Work out the finished part from the listing and answer in its coordinate system (mm). Face numbers are marked on the shaded views. A direction names the side the tool comes from. Give positions to 0.01 mm unless a question says otherwise; leave off trailing zeros. Loops run counter-clockwise (first coordinate to the right, second up) from the corner with the lowest first, then second, coordinate; pieces in that order, holes last. Notation, with made-up numbers: M 89.25,3 L 101.25,3 A18 ccw 101.25,16 Z; hole C 27,-21 d9. An arc over 180 degrees is marked long. Write item = value, one per line. Start each with the question number.
1. Consider L1, parallel to Z at x = 2, y = 57; L2, parallel to Y at x = 2, z = -19; L3, parallel to X at y = 14, z = -28. Determine where each line is inside the solid, lowest interval first. Write a range as [from, to].
2. Flat-ended cylindrical pins translate along their axes: pin 1 Ø5 at (y, z) = (19.05, -19.05) entering from -X; pin 2 Ø4 at (x, z) = (6, -10.5) entering from +Y; pin 3 Ø11 at (y, z) = (57.15, -19.05) entering from +X; pin 4 Ø1 at (y, z) = (23.5, 15.5) entering from +X. Find the tip coordinate at first contact, or state that the pin passes through.
3. Section C-C on z = 19.05 is taken. Give the number of separate pieces and of enclosed holes in the cut face, plus the area to 3 significant figures.
4. For the marked faces 1, 2 and 3, determine the directions among +Z, -Z, +X, -X, +Y, -Y from which every point of the face is accessible in a straight line to the end or side of a thin tool.
5. The mould has two halves that part along Z. Classify the marked faces 4, 5 and 6: released by +Z, released by -Z, zero draft, split by the parting line, or undercut.
6. Section A-A on x = 19 is taken. Determine the outline of the cut face in (y, z).
```python
from build123d import *

# Parameters (mm, degrees)
BOSS_EXTRUDE1_DEPTH = 35.687
FILLET1_R           = 6.35
CUT_EXTRUDE1_REACH  = 94.367
SKETCH4_R           = 4.1656
CUT_EXTRUDE2_DEPTH  = 93.366725481


with BuildPart() as part:
    # Sketch2 → Boss-Extrude1 (new, symmetric)
    with BuildSketch(Plane.XY):
        with BuildLine():
            Line((0, 0), (0, 76.2))
            Line((0, 76.2), (6.35, 76.2))
            Line((6.35, 76.2), (6.35, 14.2748))
            ThreePointArc((6.35, 14.2748), (8.67112018, 8.67112018), (14.2748, 6.35))
            Line((14.2748, 6.35), (38.1, 6.35))
            Line((38.1, 6.35), (38.1, 0))
            Line((38.1, 0), (0, 0))
        make_face()
    extrude(amount=BOSS_EXTRUDE1_DEPTH, both=True)

    # Fillet1
    fillet1_edges = [part.edges().sort_by_distance(p)[0] for p in [
        (38.1, 6.35, 0),
        (6.35, 76.2, 0),
    ]]
    fillet(fillet1_edges, radius=FILLET1_R - 0.0001)  # a hair under: the kernel refuses the full size

    # Sketch3 → Cut-Extrude1 (cut, up to next)
    with BuildSketch(Plane.XZ, mode=Mode.PRIVATE) as cut_extrude1_sk1:
        with BuildLine():
            Line((25.4, 14.8844), (12.7, 14.8844))
            ThreePointArc((12.7, 14.8844), (8.5344, 19.05), (12.7, 23.2156))
            Line((12.7, 23.2156), (25.4, 23.2156))
            ThreePointArc((25.4, 23.2156), (29.5656, 19.05), (25.4, 14.8844))
        make_face()
    cut_extrude1_tool1 = extrude(cut_extrude1_sk1.sketch, amount=-CUT_EXTRUDE1_REACH, mode=Mode.PRIVATE) & part.part
    # Sketch3 → Cut-Extrude1 (cut, up to next)
    with BuildSketch(Plane.XZ, mode=Mode.PRIVATE) as cut_extrude1_sk2:
        with BuildLine():
            Line((25.4, -23.2156), (12.7, -23.2156))
            ThreePointArc((12.7, -23.2156), (8.5344, -19.05), (12.7, -14.8844))
            Line((12.7, -14.8844), (25.4, -14.8844))
            ThreePointArc((25.4, -14.8844), (29.5656, -19.05), (25.4, -23.2156))
        make_face()
    cut_extrude1_tool2 = extrude(cut_extrude1_sk2.sketch, amount=-CUT_EXTRUDE1_REACH, mode=Mode.PRIVATE) & part.part
    add(cut_extrude1_tool1.solids().sort_by_distance((19.05, 0, 19.05))[0], mode=Mode.SUBTRACT)
    add(cut_extrude1_tool2.solids().sort_by_distance((19.05, 0, -19.05))[0], mode=Mode.SUBTRACT)

    # Sketch4 → Cut-Extrude2 (cut, through all)
    with BuildSketch(Plane.ZY):
        with Locations(Location((19.05, 57.15, 0), (0, 0, 270))):
            Circle(SKETCH4_R)
        with Locations(Location((-19.05, 19.05, 0), (0, 0, 270))):
            Circle(SKETCH4_R)
        with Locations(Location((-19.05, 57.15, 0), (0, 0, 270))):
            Circle(SKETCH4_R)
        with Locations(Location((19.05, 19.05, 0), (0, 0, 270))):
            Circle(SKETCH4_R)
    extrude(amount=-CUT_EXTRUDE2_DEPTH, mode=Mode.SUBTRACT)


solid = part.part
```
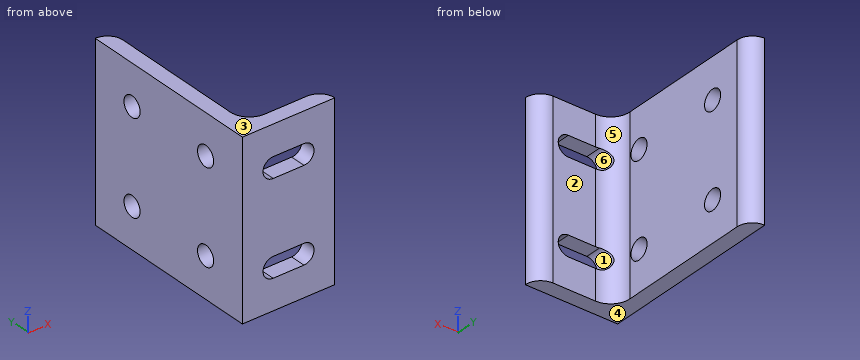
Verdict:
q1.L1 = [-35.69, -23.21], [-14.89, 14.89], [23.21, 35.69]
q1.L2 = [0, 14.88], [23.22, 52.98], [61.32, 75.88]
q1.L3 = [0, 6.35]
q2.pin_1 = through
q2.pin_2 = 74.78
q2.pin_3 = 6.35
q2.pin_4 = 6.35
q3.separate_pieces = 4
q3.enclosed_holes = 0
q3.area = 438 mm2
q4.face_1 = +Y, -Y
q4.face_2 = +Z, -Z, +X, +Y
q4.face_3 = +Z, +X, -X, +Y, -Y
q5.face_4 = released by -Z
q5.face_5 = zero draft
q5.face_6 = undercut
q6.outline = M 0,-35.69 L 6.35,-35.69 L 6.35,-23.22 L 0,-23.22 Z; M 0,-14.88 L 6.35,-14.88 L 6.35,14.88 L 0,14.88 Z; M 0,23.22 L 6.35,23.22 L 6.35,35.69 L 0,35.69 Z
